Check sheet for the drawn part. Datum: minimum x, y, z corner. Units: mm. Coordinates: 2 decimals unless noted, no trailing zeros. Loops run counter-clockwise (first coordinate to the right, second up) from the corner with the lowest first, then second, coordinate; pieces in that order, holes last. Notation, with made-up numbers: (2, -34.75) - (25, -34.75) arc R15 cw to (25, -26.75) - close; hole circle Ø7 at (8, 56). An arc over 180 degrees is marked (long way). Answer as CSV lines item,"result". Start each with the question number.
1. Cross-section at A-A (z = 23). Enter the section's corners in (x, y).
2. Gauge pin test, flat ends, axial feed: P1, Ø4, axis at x = 9.5, z = 22.5, coming from the +Y side (3 decimals); P2, Ø4, axis at y = 11, z = 29, coming from the +X side; P3, Ø1.5, axis at x = 2.5, y = 5.5, coming from the -Z side; P4, Ø7, axis at x = 6.35, y = 6.35, coming from the +Z side. Record the tip position at first contact, or that the pin passes through.
3. Release check for a two-part mould opening along Y. For the marked faces 1 and 2 record: pulls with the +Y half, pulls with the -Y half, needs draft (parallel to the pull), parting line crosses it, or undercut.
4. Material ranges on line 1 (Y direction, x = 6.35, z = 39.55); line 2 (Y direction, x = 10.5, z = 6.5) (1 decimal); line 3 (Z direction, x = 10.5, y = 4.5), recorded low to high. Write a range as [from, to].
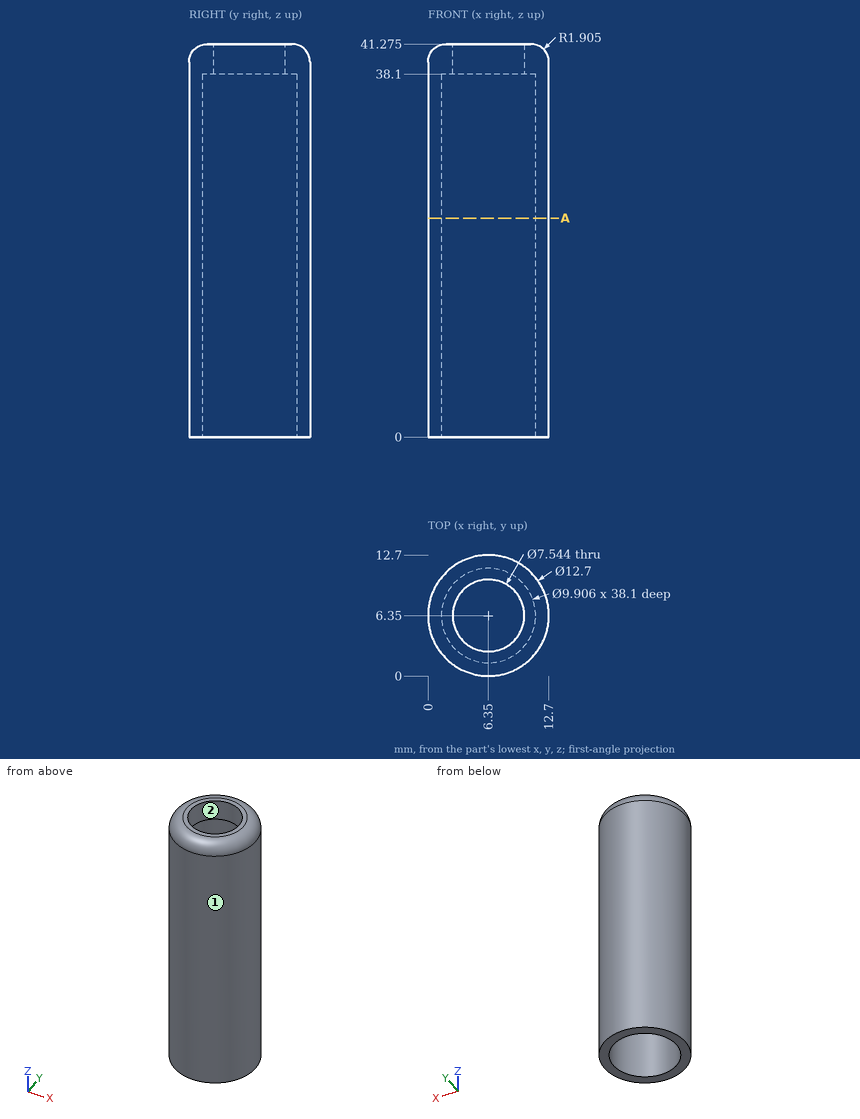
Values follow:
1,outline,"circle Ø12.7 at (6.35, 6.35); hole circle Ø9.91 at (6.35, 6.35)"
2,P1,"stops at y = 12.595"
2,P2,"stops at x = 12.12"
2,P3,"stops at z = 38.1"
2,P4,"passes through"
3,face 1,"parting line crosses it"
3,face 2,"undercut"
4,line 1,"y = [0.01, 2.58], [10.12, 12.69]"
4,line 2,"y = [1.5, 3.6], [9.1, 11.2]"
4,line 3,"z = [38.1, 41.27]"
